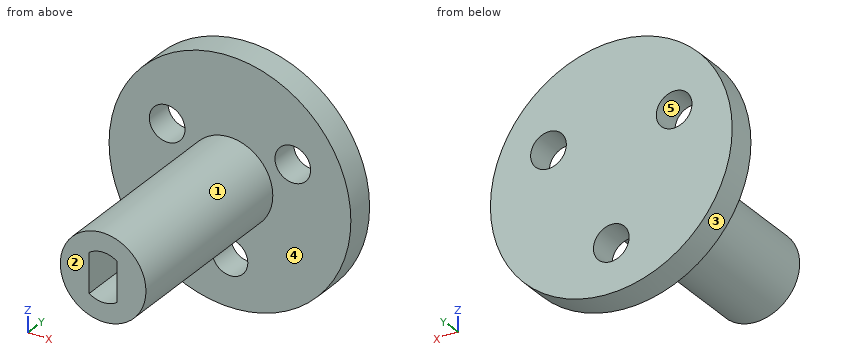
from build123d import *

# Parameters (mm, degrees)
SKETCH1_R           = 4.5
BOSS_EXTRUDE1_DEPTH = 20.32
SKETCH2_R           = 12.7
SKETCH2_R_2         = 1.875
BOSS_EXTRUDE2_DEPTH = 3
CUT_EXTRUDE1_DEPTH  = 5.842


with BuildPart() as part:
    # Sketch1 → Boss-Extrude1 (new body)
    with BuildSketch(Plane(origin=(0, 0, 0), x_dir=(1, 0, 0), z_dir=(0, 1, 0))):
        Circle(SKETCH1_R)
    extrude(amount=BOSS_EXTRUDE1_DEPTH)

    # Sketch2 → Boss-Extrude2 (add)
    with BuildSketch(Plane(origin=(0, 20.32, 0), x_dir=(1, 0, 0), z_dir=(0, 1, 0))):
        Circle(SKETCH2_R)
        with Locations((0, 7.62)):
            Circle(SKETCH2_R_2, mode=Mode.SUBTRACT)
        with Locations((6.599113577, -3.81)):
            Circle(SKETCH2_R_2, mode=Mode.SUBTRACT)
        with Locations((-6.599113577, -3.81)):
            Circle(SKETCH2_R_2, mode=Mode.SUBTRACT)
    extrude(amount=BOSS_EXTRUDE2_DEPTH)

    # Sketch3 → Cut-Extrude1 (cut)
    with BuildSketch(Plane.XZ):
        with BuildLine():
            Line((1.4605, 2.078109658), (1.4605, -2.078109658))
            ThreePointArc((1.4605, -2.078109658), (0, -2.54), (-1.4605, -2.078109658))
            Line((-1.4605, -2.078109658), (-1.4605, 2.078109658))
            ThreePointArc((-1.4605, 2.078109658), (0, 2.54), (1.4605, 2.078109658))
        make_face()
    extrude(amount=-CUT_EXTRUDE1_DEPTH, mode=Mode.SUBTRACT)


solid = part.part
Could you check a few things on this model? Use its own coordinates, in mm. Face numbers are marked on the shaded views. A direction names the side the tool comes from. Give positions to 0.01 mm unless a question says otherwise; leave off trailing zeros. Order: outer loops, then holes, each group sorted by start corner. A loop starts at its lowest first (then second) coordinate and runs counter-clockwise, first axis right, second up. Notation, with made-up numbers: (-16.75, 62) -> (-12.75, 62) arc R27 cw to (-12.75, 100) -> close; hole circle Ø4 at (28.5, 15). An arc over 180 degrees is marked (long way). Return JSON: item names as keys, results as strings.
1. Imagine slicing it at D-D on y = 5. List the corners of the cut face in (x, z) for me, then the cut area to 3 significant figures.
Answer list:
{"outline": "circle Ø9 at (0, 0); hole (-1.46, -2.08) arc R2.54 ccw to (1.46, -2.08) -> (1.46, 2.08) arc R2.54 ccw to (-1.46, 2.08) -> close", "area": "49.6 mm2"}
2. Imagine slicing it at C-C on z = 0. List the corners of the cut face in (x, y) for me, then the cut area to 3 significant figures.
Answer list:
{"outline": "(-12.7, 20.32) -> (-4.5, 20.32) -> (-4.5, 0) -> (-1.46, 0) -> (-1.46, 5.84) -> (1.46, 5.84) -> (1.46, 0) -> (4.5, 0) -> (4.5, 20.32) -> (12.7, 20.32) -> (12.7, 23.32) -> (-12.7, 23.32) -> close", "area": "242 mm2"}
3. I need wall thicknesses on line 1 (Z direction, x = 0, y = 21.7) (3 decimals); line 2 (Y direction, x = 4, z = 6.25); line 3 (X direction, y = 21.3, z = 3.81). Which ranges of each line are inside material? Lowest first, please. Write a range as from..to.
Answer list:
{"line 1": "z = -12.7..-9.495, -5.745..12.7", "line 2": "y = 20.32..23.32", "line 3": "x = -12.12..-8.47, -4.72..4.72, 8.47..12.12"}
4. Thinking about a two-plate mould opening in X: for the marked faces 3, 4 and 5, which applies, pulls with the +X half, pulls with the -X half, needs draft (parallel to the pull), parting line crosses it, or undercut?
Answer list:
{"face 3": "parting line crosses it", "face 4": "needs draft", "face 5": "undercut"}
5. For pin 1 Ø1.2 at (y, z) = (1.5, 0) entering from +X; pin 2 Ø4 at (y, z) = (20, 5) entering from +X; pin 3 Ø2 at (x, y) = (6, 18) entering from -Z; pin 4 Ø1.5 at (x, y) = (1, 14) entering from -Z, each with a flat end and sliding along its axis, tell me the tip position at first contact or that it passes through.
Answer list:
{"pin 1": "stops at x = 4.5", "pin 2": "stops at x = 12.33", "pin 3": "passes through", "pin 4": "stops at z = -4.49"}
6. Imagine slicing it at B-B on z = -7.62. List the corners of the cut face in (x, y) for me (3 decimals), then the cut area to 3 significant figures.
Answer list:
{"outline": "(-10.16, 20.32) -> (-1.875, 20.32) -> (-1.875, 23.32) -> (-10.16, 23.32) -> close; (1.875, 20.32) -> (10.16, 20.32) -> (10.16, 23.32) -> (1.875, 23.32) -> close", "area": "49.7 mm2"}
7. On a 3-axis mill with a long thin cutter (end or side, diameter ignored), from which of +Z, -Z, +X, -X, +Y, -Y can I reach the whole of each face in a straight line? I mean the marked faces 1 and 2. Say none if no direction works.
Answer list:
{"face 1": "-Y", "face 2": "+Z, -Z, +X, -X, -Y"}
8. Imagine slicing it at A-A on x = 0. List the corners of the cut face in (y, z) for me (3 decimals).
Answer list:
{"outline": "(0, -4.5) -> (20.32, -4.5) -> (20.32, -5.745) -> (23.32, -5.745) -> (23.32, 12.7) -> (20.32, 12.7) -> (20.32, 4.5) -> (0, 4.5) -> (0, 2.54) -> (5.842, 2.54) -> (5.842, -2.54) -> (0, -2.54) -> close; (20.32, -12.7) -> (23.32, -12.7) -> (23.32, -9.495) -> (20.32, -9.495) -> close"}
